Could you check a few things on this drawing? It's one solid part, dimensions in mm from its lowest x, y, z. A direction names the side the tool comes from. Round coordinates to 2 decimals unless told otherwise and drop trailing zeros. Order: outer loops, then holes, each group sorted by start corner. A loop starts at its lowest first (then second) coordinate and runs counter-clockwise, first axis right, second up. Notation, with made-up numbers: M 1.25,85.25 L 25.25,85.25 A31 ccw 25.25,118.25 Z; hole C 80,24.25 d3. An arc over 180 degrees is marked long. Answer as CSV lines item,"result". Start each with the question number.
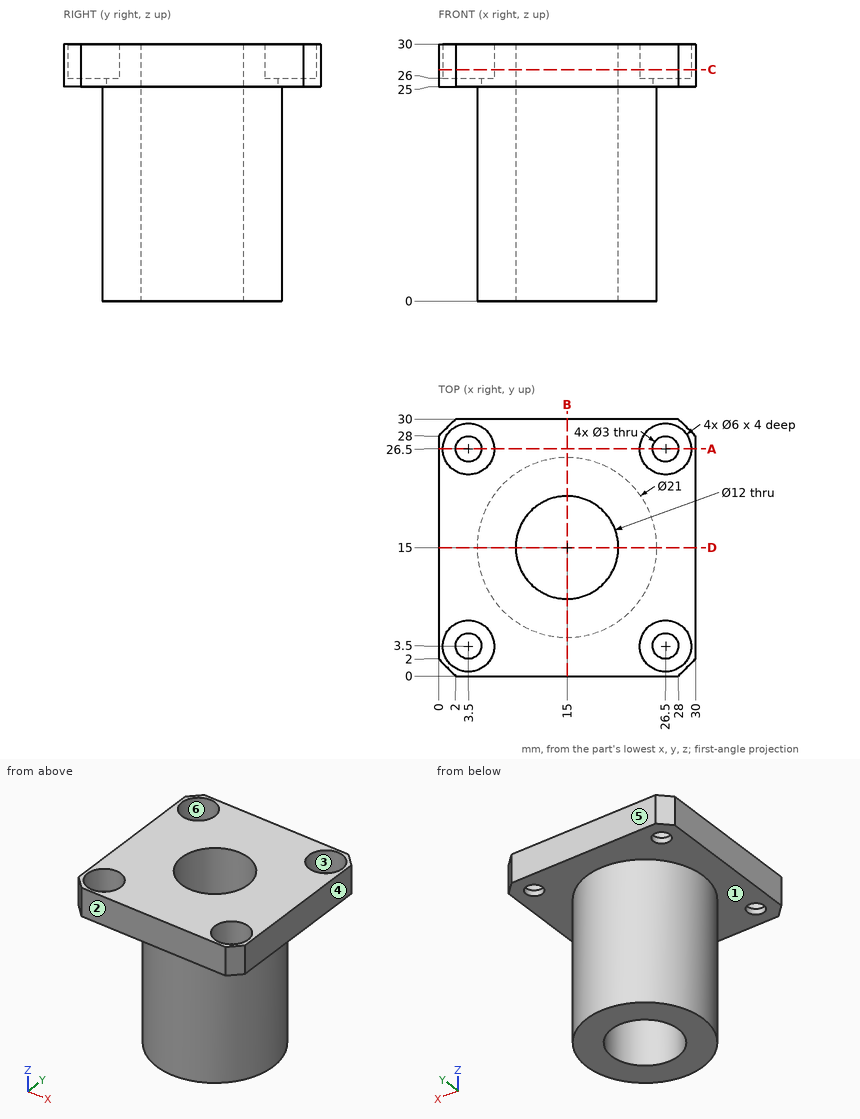
Item 1: If we section it at B-B on x = 15: Please give me the cut outline in (y, z).
Item 2: Which directions (+Z, -Z, +X, -X, +Y, -Y) give clear straight access to the entire face, cutting with the end or side of a thin tool? Please do the marked faces 1, 2 and 3.
Item 3: We'd pull the mould along Y, two halves only. Please class the marked faces 4, 5 and 6: pulls with the +Y half, pulls with the -Y half, needs draft (parallel to the pull), parting line crosses it, or undercut.
Item 4: If we section it at C-C on z = 27: Please give me the cut outline in (x, y).
Item 5: For P1, Ø9.5, axis at x = 26.5, y = 3.5, coming from the -Z side; P2, Ø4, axis at y = 8, z = 4, coming from the +X side; P3, Ø12, axis at y = 15, z = 5.5, coming from the -X side, each with a flat end and sliding along its axis, tell me the tip position at first contact or that it passes through.
Item 6: If we section it at A-A on y = 26.5: Please give me the cut outline in (x, z).
Item 7: If I drill on line 1 along Y through (x, z) = (3.5, 25.5); line 2 along Y through (x, z) = (26.5, 29.2), over which ranges is the centre line in solid material (lowest first)?
Geometry says:
1,outline,"M 0,25 L 4.5,25 L 4.5,0 L 9,0 L 9,30 L 0,30 Z; M 21,0 L 25.5,0 L 25.5,25 L 30,25 L 30,30 L 21,30 Z"
2,face 1,"-Z"
2,face 2,"+Z, -Z, +X, -X, -Y"
2,face 3,"+Z"
3,face 4,"needs draft"
3,face 5,"pulls with the +Y half"
3,face 6,"undercut"
4,outline,"M 0,2 L 2,0 L 28,0 L 30,2 L 30,28 L 28,30 L 2,30 L 0,28 Z; hole C 3.5,3.5 d6; hole C 3.5,26.5 d6; hole C 15,15 d12; hole C 26.5,3.5 d6; hole C 26.5,26.5 d6"
5,P1,"z = 25"
5,P2,"x = 24.23"
5,P3,"x = 4.5"
6,outline,"M 0,25 L 2,25 L 2,26 L 0.5,26 L 0.5,30 L 0,30 Z; M 5,25 L 25,25 L 25,26 L 23.5,26 L 23.5,30 L 6.5,30 L 6.5,26 L 5,26 Z; M 28,25 L 30,25 L 30,30 L 29.5,30 L 29.5,26 L 28,26 Z"
7,line 1,"0 to 2, 5 to 25, 28 to 30"
7,line 2,"0 to 0.5, 6.5 to 23.5, 29.5 to 30"
